```python
from build123d import *

# Parameters (mm, degrees)
PAD004_DEPTH = 20
SKETCH013_R  = 3
HOLE_DEPTH   = 25
HOLE_TIPS_R  = 3


with BuildPart() as part:
    # Sketch014 → Pad004 (new body, symmetric)
    with BuildSketch(Plane.YZ):
        Polygon((0, -35), (0, 0), (25, 0), (25, -15), (23, -15), (23, -2), (2, -2), (2, -35), align=None)
    extrude(amount=PAD004_DEPTH, both=True)

    # Sketch013 → Hole (cut)
    with BuildSketch(Plane.XZ):
        with Locations((-9.25, -22.5)):
            Circle(SKETCH013_R)
        with Locations((9.25, -22.5)):
            Circle(SKETCH013_R)
    extrude(amount=-HOLE_DEPTH, mode=Mode.SUBTRACT)

    # Hole tips → Hole tip 1 section 0
    with BuildSketch(Plane.XZ.offset(-25), mode=Mode.PRIVATE) as hole_tip_1_s0:
        with Locations((-9.25, -22.5)):
            Circle(HOLE_TIPS_R)
    loft([hole_tip_1_s0.sketch, Vertex(-9.25, 26.802582, -22.5)], mode=Mode.SUBTRACT)

    # Hole tips → Hole tip 2 section 0
    with BuildSketch(Plane.XZ.offset(-25), mode=Mode.PRIVATE) as hole_tip_2_s0:
        with Locations((9.25, -22.5)):
            Circle(HOLE_TIPS_R)
    loft([hole_tip_2_s0.sketch, Vertex(9.25, 26.802582, -22.5)], mode=Mode.SUBTRACT)


with BuildPart() as part_1:
    # Body009 placement: moved
    add(part.part.moved(Location((0, 83, 0))))


with BuildPart() as part_2:
    # Clone008 placement: moved
    add(part_1.part.moved(Location((0, -83, 0))))


with BuildPart() as part_3:
    # Body011 placement: moved
    add(part_2.part.moved(Location((-225, 83, 450))))


solid = part_3.part
```
The listing builds one solid part. Answer for the finished solid, in the listing's coordinates (mm). A direction names the side the tool comes from. Coordinates: 2 decimals unless noted, no trailing zeros. Write each loop counter-clockwise with the first axis right and the second up, starting at its lowest first coordinate (ties: lowest second). Pieces come first, ordered by that corner, then holes.
Q1. The mould has two halves that part along Y. Classify faces 1 (the flat face through (-225, 85, 432)), 2 (the flat face through (-205, 84, 440)), 3 (the flat face through (-225, 83, 432)): released by +Y, released by -Y, zero draft, split by the parting line, or undercut.
Returned:
face 1: undercut
face 2: zero draft
face 3: released by -Y
Q2. Which of the six approach directions +Z, -Z, +X, -X, +Y, -Y give full straight-line access (tool end or side, diameter ignored) to faces 4 (the cylindrical face through (-218.131, 83.986, 425.675)), 5 (the flat face through (-225, 107, 435)), 6 (the flat face through (-225, 106, 441))?
Returned:
face 4: +Y, -Y
face 5: -Z, +X, -X, +Y
face 6: -Z, +X, -X
Q3. Find the intervals of material crossed by line 1 along X through (y, z) = (84.6, 427.5); line 2 along Z through (x, y) = (-215.75, 83.8); line 3 along Y through (x, z) = (-228.5, 445), in increasing order.
Returned:
line 1: x = -245 to -237.25, -231.25 to -218.75, -212.75 to -205
line 2: z = 415 to 424.5, 430.5 to 450
line 3: y = 83 to 85, 106 to 108
Q4. Section B-B, the plane x = -234.25 is taken. Write down the section's boundary in (y, z), then the cut area to 3 significant figures.
Returned:
outline: (83, 415) - (85, 415) - (85, 424.5) - (83, 424.5) - close; (83, 430.5) - (85, 430.5) - (85, 448) - (106, 448) - (106, 435) - (108, 435) - (108, 450) - (83, 450) - close
area: 130 mm2
Q5. Section A-A, the plane z = 427.5 is taken. Write down the section's boundary in (x, y).
Returned:
outline: (-245, 83) - (-237.25, 83) - (-237.25, 85) - (-245, 85) - close; (-231.25, 83) - (-218.75, 83) - (-218.75, 85) - (-231.25, 85) - close; (-212.75, 83) - (-205, 83) - (-205, 85) - (-212.75, 85) - close
Q6. Given P1, Ø5, axis at x = -216.5, z = 428.5, coming from the +Y side; P2, Ø5, axis at x = -211.5, y = 87, coming from the -Z side; P3, Ø6.5, axis at x = -222, y = 90.5, coming from the -Z side; P4, Ø1, axis at x = -222.5, y = 107.5, coming from the -Z side, each flat-ended and moving along its own axis, determine where each tip first touches the part or whether it passes through.
Returned:
P1: stops at y = 85
P2: stops at z = 415
P3: stops at z = 448
P4: stops at z = 435
Q7. Section D-D, the plane x = -211 is taken. Write down the section's boundary in (y, z), then the cut area to 3 significant figures.
Returned:
outline: (83, 415) - (85, 415) - (85, 448) - (106, 448) - (106, 435) - (108, 435) - (108, 450) - (83, 450) - close
area: 142 mm2
Q8. Section C-C, the plane z = 443.5 is taken. Write down the section's boundary in (x, y), then the cut area to 3 significant figures.
Returned:
outline: (-245, 83) - (-205, 83) - (-205, 85) - (-245, 85) - close; (-245, 106) - (-205, 106) - (-205, 108) - (-245, 108) - close
area: 160 mm2
